Geometry: final body of the model. Coordinates: model frame, mm. A direction names the side the tool comes from. Round coordinates to 2 decimals unless told otherwise and drop trailing zeros. Loops run counter-clockwise (first coordinate to the right, second up) from the corner with the lowest first, then second, coordinate; pieces in that order, holes last. Notation, with made-up numbers: M 22,21.5 L 47,21.5 A25 cw 47,59.5 Z; hole C 51.25,-12 d11. An arc over 180 degrees is marked long. Answer as a JSON object with one key per item and string values.
from build123d import *

# Parameters (mm, degrees)
SKETCH1_W           = 49
SKETCH1_H           = 101
BOSS_EXTRUDE1_DEPTH = 1.5
SKETCH2_W           = 54
SKETCH2_H           = 106
SKETCH2_W_2         = 49
SKETCH2_H_2         = 101
BOSS_EXTRUDE2_DEPTH = 4
SKETCH3_W           = 5.5
SKETCH3_H           = 15
BOSS_EXTRUDE3_DEPTH = 5
SKETCH4_R           = 1.75
CUT_EXTRUDE1_DEPTH  = 4.25
SKETCH5_R           = 1.75
CUT_EXTRUDE2_DEPTH  = 4.25
SKETCH6_W           = 14.5
SKETCH6_H           = 7.3
CUT_EXTRUDE3_DEPTH  = 60.690870324
SKETCH7_W           = 13.8
SKETCH7_H           = 6
CUT_EXTRUDE4_DEPTH  = 60.690870324
FILLET1_R           = 3
CUT_EXTRUDE5_DEPTH  = 60.690870324
FILLET2_R           = 1.5875


with BuildPart() as part:
    # Sketch1 → Boss-Extrude1 (new body)
    with BuildSketch(Plane(origin=(0, 0, 0), x_dir=(1, 0, 0), z_dir=(0, 1, 0))):
        Rectangle(SKETCH1_W, SKETCH1_H)
    extrude(amount=BOSS_EXTRUDE1_DEPTH)

    # Sketch2 → Boss-Extrude2 (add)
    with BuildSketch(Plane(origin=(0, 0, 0), x_dir=(1, 0, 0), z_dir=(0, 1, 0))):
        Rectangle(SKETCH2_W, SKETCH2_H)
        Rectangle(SKETCH2_W_2, SKETCH2_H_2, mode=Mode.SUBTRACT)
    extrude(amount=BOSS_EXTRUDE2_DEPTH)

    # Sketch3 → Boss-Extrude3 (add)
    with BuildSketch(Plane(origin=(0, 0, 0), x_dir=(1, 0, 0), z_dir=(0, 1, 0))):
        with BuildLine():
            Line((-24.5, -30.741687605), (-24.5, -34.058312395))
            ThreePointArc((-24.5, -34.058312395), (-19, -32.4), (-24.5, -30.741687605))
        make_face()
        with Locations((-21.75, 0)):
            Rectangle(SKETCH3_W, SKETCH3_H)
        with BuildLine():
            Line((-24.5, -46.403337045), (-24.5, -49.396662955))
            ThreePointArc((-24.5, -49.396662955), (-24.021320344, -50.021320344), (-23.396662955, -50.5))
            Line((-23.396662955, -50.5), (-20.403337045, -50.5))
            ThreePointArc((-20.403337045, -50.5), (-19.778679656, -45.778679656), (-24.5, -46.403337045))
        make_face()
    boss_extrude3 = extrude(amount=BOSS_EXTRUDE3_DEPTH)

    # Mirror1: Boss-Extrude3 across plane
    add(boss_extrude3.mirror(Plane(origin=(0, 0, 0), x_dir=(0, 0, 1), z_dir=(1, 0, 0))))

    # Sketch4 → Cut-Extrude1 (cut)
    with BuildSketch(Plane(origin=(0, 5, 0), x_dir=(1, 0, 0), z_dir=(0, 1, 0))):
        with Locations(Location((-21.9, -47.9, 0), (0, 0, 270))):
            Circle(SKETCH4_R)
        with Locations(Location((21.9, -47.9, 0), (0, 0, 270))):
            Circle(SKETCH4_R)
    extrude(amount=-CUT_EXTRUDE1_DEPTH, mode=Mode.SUBTRACT)

    # Sketch5 → Cut-Extrude2 (cut)
    with BuildSketch(Plane(origin=(0, 5, 0), x_dir=(1, 0, 0), z_dir=(0, 1, 0))):
        with Locations(Location((-22, -32.4, 0), (0, 0, 270))):
            Circle(SKETCH5_R)
        with Locations(Location((22, -32.4, 0), (0, 0, 270))):
            Circle(SKETCH5_R)
    extrude(amount=-CUT_EXTRUDE2_DEPTH, mode=Mode.SUBTRACT)

    # Sketch6 → Cut-Extrude3 (cut, through all)
    with BuildSketch(Plane(origin=(0, 0, 0), x_dir=(1, 0, 0), z_dir=(0, 1, 0))):
        with Locations((-1.75, -48.65)):
            Rectangle(SKETCH6_W, SKETCH6_H)
    extrude(amount=CUT_EXTRUDE3_DEPTH, mode=Mode.SUBTRACT)

    # Sketch7 → Cut-Extrude4 (cut, through all)
    with BuildSketch(Plane(origin=(0, 0, 0), x_dir=(1, 0, 0), z_dir=(0, 1, 0))):
        with Locations((12.4, -45.7)):
            Rectangle(SKETCH7_W, SKETCH7_H)
    extrude(amount=CUT_EXTRUDE4_DEPTH, mode=Mode.SUBTRACT)

    # Fillet1
    fillet1_edges = [part.edges().sort_by_distance(p)[0] for p in [
        (-27, 2, 53),
        (27, 2, 53),
        (27, 2, -53),
        (-27, 2, -53),
    ]]
    fillet(fillet1_edges, radius=FILLET1_R)

    # Sketch9 → Cut-Extrude5 (cut, through all)
    with BuildSketch(Plane(origin=(0, 0, 0), x_dir=(1, 0, 0), z_dir=(0, 1, 0))):
        with BuildLine():
            Line((-7.814445172, -44.472009202), (4.314445172, -44.472009202))
            ThreePointArc((4.314445172, -44.472009202), (4.582924338, -44.36080149), (4.69413205, -44.092322323))
            Line((4.69413205, -44.092322323), (4.69413205, -43.905796609))
            ThreePointArc((4.69413205, -43.905796609), (5.159832268, -42.781496827), (6.28413205, -42.315796609))
            Line((6.28413205, -42.315796609), (18.263585731, -42.315796609))
            ThreePointArc((18.263585731, -42.315796609), (19.387885513, -42.781496827), (19.853585731, -43.905796609))
            Line((19.853585731, -43.905796609), (19.853585731, -47.487814705))
            ThreePointArc((19.853585731, -47.487814705), (19.387885513, -48.612114487), (18.263585731, -49.077814705))
            Line((18.263585731, -49.077814705), (7.489445172, -49.077814705))
            ThreePointArc((7.489445172, -49.077814705), (6.366913156, -49.54278269), (5.901945172, -50.665314705))
            Line((5.901945172, -50.665314705), (5.901945172, -53))
            Line((5.901945172, -53), (-9.401945172, -53))
            Line((-9.401945172, -53), (-9.401945172, -46.059509202))
            ThreePointArc((-9.401945172, -46.059509202), (-8.936977187, -44.936977187), (-7.814445172, -44.472009202))
        make_face()
    extrude(amount=CUT_EXTRUDE5_DEPTH, mode=Mode.SUBTRACT)

    # Fillet2
    # the kernel refuses this fillet: 1.5875 mm, written as the material it adds along each edge
    with BuildSketch(Plane(origin=(20.403337045, 1.5, 50.5), x_dir=(-0.6349026308265473, 0, -0.7725921623790454), z_dir=(0, 1, 0))) as fillet2_piece_1:
        with BuildLine():
            CenterArc((3.087304614, 1.256456201), FILLET2_R, 140.587236848, 91.735718276)
            Line((1.860814556, 2.264364128), (0, 0))
            ThreePointArc((0, 0), (1.058504375, 0.192943091), (2.11700875, 0))
        make_face()
    extrude(amount=2.5)
    with BuildSketch(Plane(origin=(24.5, 1.5, 46.403337045), x_dir=(-0.8047683960868028, 0, -0.5935889391320183), z_dir=(0, 1, 0))) as fillet2_piece_2:
        with BuildLine():
            CenterArc((3.045104664, -1.45404326), FILLET2_R, 113.661459125, 102.750646884)
            Line((1.767534835, -2.396365701), (0, 0))
            ThreePointArc((0, 0), (1.203995254, -0.252201713), (2.407990509, 0))
        make_face()
    extrude(amount=2.5)
    with BuildSketch(Plane(origin=(24.5, 1.5, 34.058312395), x_dir=(-0.8294476443903582, 0, 0.5585844656050558), z_dir=(0, 1, 0)), Plane(origin=(-24.5, 1.5, 30.741687605), x_dir=(0.8294476443903578, 0, -0.5585844656050566), z_dir=(0, 1, 0))) as fillet2_piece_3:
        with BuildLine():
            CenterArc((2.901742174, 1.466820617), FILLET2_R, 146.042039471, 101.473230821)
            Line((1.584994038, 2.353573457), (0, 0))
            ThreePointArc((0, 0), (1.147311568, 0.228055526), (2.294623136, 0))
        make_face()
    extrude(amount=2.5)
    with BuildSketch(Plane(origin=(24.5, 1.5, 30.741687605), x_dir=(-0.8294476443903573, 0, -0.5585844656050574), z_dir=(0, 1, 0)), Plane(origin=(-24.5, 1.5, 34.058312395), x_dir=(0.8294476443903588, 0, 0.5585844656050553), z_dir=(0, 1, 0))) as fillet2_piece_4:
        with BuildLine():
            CenterArc((2.901742174, -1.466820617), FILLET2_R, 112.484729709, 101.473230821)
            Line((1.584994038, -2.353573457), (0, 0))
            ThreePointArc((0, 0), (1.147311568, -0.228055526), (2.294623136, 0))
        make_face()
    extrude(amount=2.5)
    with BuildSketch(Plane(origin=(24.5, 1.5, -7.5), x_dir=(-1, 0, 0), z_dir=(0, 1, 0)), Plane(origin=(-24.5, 1.5, 7.5), x_dir=(1, 0, 0), z_dir=(0, 1, 0))) as fillet2_piece_5:
        with BuildLine():
            CenterArc((FILLET2_R, -FILLET2_R), FILLET2_R, 90, 90)
            Line((0, -FILLET2_R), (0, 0))
            Line((0, 0), (FILLET2_R, 0))
        make_face()
    extrude(amount=2.5)
    with BuildSketch(Plane(origin=(24.5, 1.5, 7.5), x_dir=(-1, 0, 0), z_dir=(0, 1, 0)), Plane(origin=(24.5, 1.5, -50.5), x_dir=(-1, 0, 0), z_dir=(0, 1, 0)), Plane(origin=(-24.5, 1.5, -50.5), x_dir=(0, 0, 1), z_dir=(0, 1, 0)), Plane(origin=(-24.5, 1.5, -7.5), x_dir=(1, 0, 0), z_dir=(0, 1, 0))) as fillet2_piece_6:
        with BuildLine():
            CenterArc((FILLET2_R, FILLET2_R), FILLET2_R, 180, 90)
            Line((0, FILLET2_R), (0, 0))
            Line((0, 0), (FILLET2_R, 0))
        make_face()
    extrude(amount=2.5)
    with BuildSketch(Plane(origin=(-20.403337045, 1.5, 50.5), x_dir=(1, 0, 0), z_dir=(0, 1, 0))) as fillet2_piece_7:
        with BuildLine():
            CenterArc((2.97770851, 1.5875), FILLET2_R, 167.249353116, 102.750646884)
            ThreePointArc((1.429356531, 1.937874659), (0.917642234, 0.819233183), (0, 0))
            Line((0, 0), (2.97770851, 0))
        make_face()
    extrude(amount=2.5)
    with BuildSketch(Plane(origin=(-24.5, 1.5, 46.403337045), x_dir=(0.8047683960868005, 0, -0.5935889391320214), z_dir=(0, 1, 0))) as fillet2_piece_8:
        with BuildLine():
            CenterArc((3.045104664, 1.45404326), FILLET2_R, 143.587893991, 102.750646884)
            Line((1.767534835, 2.396365701), (0, 0))
            ThreePointArc((0, 0), (1.203995254, 0.252201713), (2.407990509, 0))
        make_face()
    extrude(amount=2.5)


solid = part.part
1) Section query D-D (y = 2.25). Count the separate pieces of the cut face and the enclosed holes in it, and give its area (3 significant figures).
Results:
{"separate pieces": "1", "enclosed holes": "6", "area": "975 mm2"}
2) Section query B-B (z = 32.4). Return the cut outline in (x, y).
Results:
{"outline": "M -27,0 L 27,0 L 27,4 L 24.5,4 L 24.5,5 L 23.75,5 L 23.75,0.75 L 20.25,0.75 L 20.25,5 L 19,5 L 19,1.5 L -19,1.5 L -19,5 L -20.25,5 L -20.25,0.75 L -23.75,0.75 L -23.75,5 L -24.5,5 L -24.5,4 L -27,4 Z"}
3) Section query C-C (x = -12.5). Return the cut outline in (y, z), and give its area (4 significant figures).
Results:
{"outline": "M 0,-53 L 4,-53 L 4,-50.5 L 1.5,-50.5 L 1.5,50.5 L 4,50.5 L 4,53 L 0,53 Z", "area": "171.5 mm2"}
4) Reachability of faces 5 (the flat face through (24.5, 3, 19)), 6 (the flat face through (15, 2, 53)) from +Z, -Z, +X, -X, +Y, -Y: full face, straight path, thin tool, end or side. Return the list, or none.
Results:
{"face 5": "+Y", "face 6": "+Z, +X, -X, +Y, -Y"}
5) Pull-direction query (X, two-part tool) for faces 1 (the flat face through (-20.6, 5, 33.7)), 2 (the cylindrical face through (-21.82, 2.9, 46.15)), 3 (the flat face through (22, 0.75, 48)), 4 (the cylindrical face through (-26.14, 2.03, -52.1)); classes: +X half, -X half, draft (parallel to the pull), parting line (faces both ways), or undercut.
Results:
{"face 1": "draft", "face 2": "undercut", "face 3": "undercut", "face 4": "-X half"}
6) Pin query (flat end, axial travel): P1, Ø0.8, axis at y = 4.5, z = 33, coming from the -X side; P2, Ø4, axis at x = 11.5, z = -32.5, coming from the +Y side; P3, Ø3, axis at x = -1.5, y = 2.5, coming from the +Z side. Return the tip coordinate at first contact, or that it passes through.
Results:
{"P1": "x = -24.5", "P2": "y = 1.5", "P3": "z = 44.47"}
7) Ray query, line 1 (X direction, y = 1.75, z = 32.4); line 2 (Z direction, x = 10.5, y = 1.65); line 3 (Z direction, x = -23.5, y = 4.15). Return the intervals inside material, ascending.
Results:
{"line 1": "-27 to -23.75, -20.25 to -19, 19 to 20.25, 23.75 to 27", "line 2": "-53 to -50.5, 50.5 to 53", "line 3": "-7.5 to 7.5, 29.8 to 31.5, 33.3 to 35, 45.36 to 47.19, 48.61 to 50.44"}
8) Section query A-A (x = 15.5). Return the cut outline in (y, z).
Results:
{"outline": "M 0,-53 L 4,-53 L 4,-50.5 L 1.5,-50.5 L 1.5,42.32 L 0,42.32 Z; M 0,49.08 L 1.5,49.08 L 1.5,50.5 L 4,50.5 L 4,53 L 0,53 Z"}
